Can you work these out from the model? Positions are in its coordinate system, mm. Face numbers are marked on the shaded views. A direction names the side the tool comes from. Give positions to 0.01 mm unless a question says otherwise; leave off trailing zeros. Loops run counter-clockwise (first coordinate to the right, second up) from the corner with the lowest first, then second, coordinate; pieces in that order, holes last. Notation, with made-up numbers: (71, 26.25) - (93, 26.25) arc R33 cw to (93, 56.25) - close; hole circle Ø4 at (25, -7). An arc over 180 degrees is marked (long way). Answer as a JSON object with one key per item and string values.
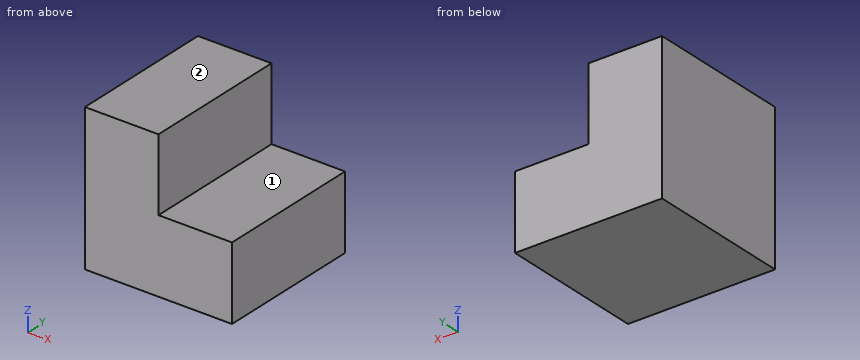
```python
from build123d import *

# Parameters (mm, degrees)
F1_DEPTH = 100


# Not quite as in the source:
# - a feature names something its author has since deleted; it is built from what else it names


with BuildPart() as f1:
    # F0 (on Front) → F1 (new body)
    with BuildSketch(Plane.XZ):
        Polygon((50, 115.3164558689), (0, 115.3164558689), (0, 15.3164558689), (100, 15.3164558689), (100, 65.5276626348), (50, 65.5276626348), align=None)
    extrude(amount=-F1_DEPTH)


solid = f1.part
```
1) Which directions (+Z, -Z, +X, -X, +Y, -Y) give clear straight access to the entire face, cutting with the end or side of a thin tool? Please do the marked faces 1 and 2.
Check sheet entries:
{"face 1": "+Z, +X, +Y, -Y", "face 2": "+Z, +X, -X, +Y, -Y"}
2) Imagine slicing it at A-A on y = 47.5. Write out the boundary of the cut face in (x, z).
Check sheet entries:
{"outline": "(0, 15.32) - (100, 15.32) - (100, 65.53) - (50, 65.53) - (50, 115.32) - (0, 115.32) - close"}
3) Imagine slicing it at B-B on z = 94. Write out the boundary of the cut face in (x, y), and give its area (3 significant figures).
Check sheet entries:
{"outline": "(0, 0) - (50, 0) - (50, 100) - (0, 100) - close", "area": "5,000 mm2"}
4) I'm going to push flat-ended pins straight in: P1, Ø3, axis at x = 80, y = 62, coming from the +Z side; P2, Ø15, axis at y = 45, z = 98.5, coming from the +X side. Where does each tip first touch, or does it pass through?
Check sheet entries:
{"P1": "z = 65.53", "P2": "x = 50"}
5) I need wall thicknesses on L1, parallel to X at y = 88.5, z = 111.5; L2, parallel to Z at x = 93, y = 44. Which ranges of each line are inside material? Lowest first, please.
Check sheet entries:
{"L1": "0 to 50", "L2": "15.32 to 65.53"}
6) Imagine slicing it at C-C on x = 64. Write out the boundary of the cut face in (y, z).
Check sheet entries:
{"outline": "(0, 15.32) - (100, 15.32) - (100, 65.53) - (0, 65.53) - close"}
